Check sheet for the modelled part. Datum: model origin and axes. Units: mm. A direction names the side the tool comes from. Round coordinates to 2 decimals unless told otherwise and drop trailing zeros. Loops run counter-clockwise (first coordinate to the right, second up) from the corner with the lowest first, then second, coordinate; pieces in that order, holes last. Notation, with made-up numbers: (-24.5, 0) -> (16.5, 0) arc R14 ccw to (16.5, 5) -> close; hole circle Ø11 at (-1, -12.75). An arc over 180 degrees is marked (long way). One line per question, with ' | ' between items.
```python
from build123d import *

# Parameters (mm, degrees)
ESQUISSE1_W                  = 16.3
ESQUISSE1_H                  = 12
BOSS_EXTRU_1_DEPTH           = 10.7
ENL_V_MAT_EXTRU_1_DEPTH      = 9
ESQUISSE4_W                  = 5.6
ESQUISSE4_H                  = 3.1
BOSS_EXTRU_2_DEPTH           = 8.8
CHANFREIN1_SIZE              = 0.2
CONG_1_R                     = 0.1
ESQUISSE5_W                  = 1.55
ESQUISSE5_H                  = 0.3
BOSS_EXTRU_3_DEPTH           = 4.3
BOSS_EXTRU_4_DEPTH           = 2.6
BOSS_EXTRU_4_DRAFT           = -15
BOSS_EXTRU_4_PROFILE_2_DEPTH = 2.6
BOSS_EXTRU_4_PROFILE_2_DRAFT = -15
CONG_3_R                     = 0.15


with BuildPart() as part:
    # Esquisse1 → Boss.-Extru.1 (new body)
    with BuildSketch(Plane(origin=(0, 0, 0), x_dir=(1, 0, 0), z_dir=(0, 1, 0))):
        with Locations((-8.15, 6)):
            Rectangle(ESQUISSE1_W, ESQUISSE1_H)
    extrude(amount=BOSS_EXTRU_1_DEPTH)

    # Esquisse2 → Enlèv. mat.-Extru.1 (cut)
    with BuildSketch(Plane.ZY.offset(16.3)):
        Polygon((-8.6, 9.25), (-10.2, 7.65), (-10.2, 1.65), (-1.8, 1.65), (-1.8, 7.65), (-3.4, 9.25), align=None)
    extrude(amount=-ENL_V_MAT_EXTRU_1_DEPTH, mode=Mode.SUBTRACT)

    # Esquisse4 → Boss.-Extru.2 (add)
    with BuildSketch(Plane.ZY.offset(7.3)):
        with Locations((-6, 5.4)):
            Rectangle(ESQUISSE4_W, ESQUISSE4_H)
    extrude(amount=BOSS_EXTRU_2_DEPTH)

    # Chanfrein1
    chanfrein1_edges = [part.edges().sort_by_distance(p)[0] for p in [
        (-16.3, 4.65, -10.2),
        (-16.3, 1.65, -6),
        (-16.3, 4.65, -1.8),
        (-16.3, 8.45, -2.6),
        (-16.3, 9.25, -6),
        (-16.3, 8.45, -9.4),
        (-11.7, 6.95, -8.8),
        (-11.7, 3.85, -8.8),
        (-11.7, 3.85, -3.2),
        (-11.7, 6.95, -3.2),
        (-16.1, 5.4, -8.8),
        (-16.1, 3.85, -6),
        (-16.1, 5.4, -3.2),
        (-16.1, 6.95, -6),
    ]]
    chamfer(chanfrein1_edges, length=CHANFREIN1_SIZE)

    # Congé1
    cong_1_edges = [part.edges().sort_by_distance(p)[0] for p in [
        (-16.3, 10.7, -6),
        (-8.15, 10.7, 0),
        (-16.3, 0, -6),
        (-8.15, 10.7, -12),
        (-16.3, 5.35, 0),
        (-16.3, 5.35, -12),
    ]]
    fillet(cong_1_edges, radius=CONG_1_R)

    # Esquisse5 → Boss.-Extru.3 (add)
    with BuildSketch(Plane.XZ):
        with Locations((-6.025, -0.15)):
            Rectangle(ESQUISSE5_W, ESQUISSE5_H)
        with Locations((-6.025, -11.85)):
            Rectangle(ESQUISSE5_W, ESQUISSE5_H)
    extrude(amount=BOSS_EXTRU_3_DEPTH)


with BuildPart() as boss_extru_4_tool:
    # Esquisse6 → Boss.-Extru.4 (with draft: the straight prism first)
    with BuildSketch(Plane(origin=(0, -1.55, 0), x_dir=(1, 0, 0), z_dir=(0, 1, 0))):
        with BuildLine():
            ThreePointArc((-6.8, 0.85), (-7.5, 0.15), (-6.8, -0.55))
            Line((-6.8, -0.55), (-5.25, -0.55))
            ThreePointArc((-5.25, -0.55), (-4.55, 0.15), (-5.25, 0.85))
            Line((-5.25, 0.85), (-6.8, 0.85))
        make_face()
    extrude(amount=-BOSS_EXTRU_4_DEPTH)
    # Boss.-Extru.4: the draft: its side faces are tilted about the plane it starts from
    boss_extru_4_sides = [boss_extru_4_tool.faces().sort_by_distance(p)[0] for p in [
        (-6.025, -2.85, 0.55),
        (-4.55, -2.85, -0.15),
        (-6.025, -2.85, -0.85),
        (-7.5, -2.85, -0.15),
    ]]
    draft(boss_extru_4_sides, Plane(origin=(0, -1.55, 0), x_dir=(1, 0, 0), z_dir=(0, 1, 0)), BOSS_EXTRU_4_DRAFT)


with BuildPart() as part_1:
    add(part.part)

    # Boss.-Extru.4: add boss_extru_4_tool
    add(boss_extru_4_tool.part)


with BuildPart() as boss_extru_4_profile_2_tool:
    # Esquisse6 → Boss.-Extru.4 profile 2 (with draft: the straight prism first)
    with BuildSketch(Plane(origin=(0, -1.55, 0), x_dir=(1, 0, 0), z_dir=(0, 1, 0))):
        with BuildLine():
            ThreePointArc((-6.8, 12.55), (-7.5, 11.85), (-6.8, 11.15))
            Line((-6.8, 11.15), (-5.25, 11.15))
            ThreePointArc((-5.25, 11.15), (-4.55, 11.85), (-5.25, 12.55))
            Line((-5.25, 12.55), (-6.8, 12.55))
        make_face()
    extrude(amount=-BOSS_EXTRU_4_PROFILE_2_DEPTH)
    # Boss.-Extru.4 profile 2: the draft: its side faces are tilted about the plane it starts from
    boss_extru_4_profile_2_sides = [boss_extru_4_profile_2_tool.faces().sort_by_distance(p)[0] for p in [
        (-7.5, -2.85, -11.85),
        (-6.025, -2.85, -11.15),
        (-4.55, -2.85, -11.85),
        (-6.025, -2.85, -12.55),
    ]]
    draft(boss_extru_4_profile_2_sides, Plane(origin=(0, -1.55, 0), x_dir=(1, 0, 0), z_dir=(0, 1, 0)), BOSS_EXTRU_4_PROFILE_2_DRAFT)


with BuildPart() as part_2:
    add(part_1.part)

    # Boss.-Extru.4 profile 2: add boss_extru_4_profile_2_tool
    add(boss_extru_4_profile_2_tool.part)

    # Congé3
    cong_3_edges = [part_2.edges().sort_by_distance(p)[0] for p in [
        (-6.8, -4.3, -0.15),
        (-6.025, -4.3, -0.3),
        (-5.25, -4.3, -0.15),
        (-6.025, -4.3, 0),
        (-6.025, -4.3, -12),
        (-5.25, -4.3, -11.85),
        (-6.025, -4.3, -11.7),
        (-6.8, -4.3, -11.85),
    ]]
    fillet(cong_3_edges, radius=CONG_3_R - 0.0001)  # a hair under: the kernel refuses the full size


solid = part_2.part
```
(1) Set-up check for faces 4 (the face through (-6.04, -2.56, -11.42)), 5 (the face through (-8, 4, -12)), 6 (the face through (-8, 10.7, -6)), 7 (the face through (-4.894, -2.832, -0.142)), 8 (the face through (-11.76, 8.44, -2.59)): record each of +Z, -Z, +X, -X, +Y, -Y from which the full face is reachable in a straight line by a thin tool's end or side.
Answer:
face 4: +X, -X, -Y | face 5: -Z, +X, -X, +Y | face 6: +Z, -Z, +X, -X, +Y | face 7: +X, -Y | face 8: -X
(2) Go/stop test with flat-tipped pins: pin 1 (6.5 mm diameter, centred on x = -9.5, y = 5, fed in from +Z); pin 2 (6 mm diameter, centred on x = -5, z = -6, fed in from -Y); pin 3 (3 mm diameter, centred on y = 5.5, z = -7, fed in from -X). Record where each tip stops, or that it passes through.
Answer:
pin 1: stops at z = 0 | pin 2: stops at y = 0 | pin 3: stops at x = -16.1
(3) Scan lines: probe 1 along Y at (x, z) = (-14, -6.5); probe 2 along Z at (x, y) = (-15.5, 3.25). Record each from-to range of solid material in increasing order.
Answer:
probe 1: y = 0 to 1.65, 3.85 to 6.95, 9.25 to 10.7 | probe 2: z = -12 to -10.2, -1.8 to 0
(4) Sectioned sample at B-B, the plane x = -3. Record the cut outline in (y, z).
Answer:
outline: (0, -12) -> (10.6, -12) arc R0.1 ccw to (10.7, -11.9) -> (10.7, -0.1) arc R0.1 ccw to (10.6, 0) -> (0, 0) -> close
(5) Sectioned sample at A-A, the plane z = -8.25. Record the cut outline in (x, y).
Answer:
outline: (-16.3, 0.1) arc R0.1 ccw to (-16.2, 0) -> (0, 0) -> (0, 10.7) -> (-16.2, 10.7) arc R0.1 ccw to (-16.3, 10.6) -> (-16.3, 9.45) -> (-16.1, 9.25) -> (-7.3, 9.25) -> (-7.3, 6.95) -> (-15.9, 6.95) -> (-16.1, 6.75) -> (-16.1, 4.05) -> (-15.9, 3.85) -> (-7.3, 3.85) -> (-7.3, 1.65) -> (-16.1, 1.65) -> (-16.3, 1.45) -> close
(6) Mould release check, pull along Y, two halves, no side actions. Record for faces 1 (the face through (-6.01, -2.56, -12.28)), 2 (the face through (-12, 6.95, -6)), 3 (the face through (-8, 4, 0)): +Y half, -Y half, draft (parallel to the pull), parting line (faces both ways), or undercut.
Answer:
face 1: -Y half | face 2: undercut | face 3: draft
(7) Sectioned sample at C-C, the plane z = -2.75. Record the cut outline in (x, y), and give its area (3 significant figures).
Answer:
outline: (-16.3, 0.1) arc R0.1 ccw to (-16.2, 0) -> (0, 0) -> (0, 10.7) -> (-16.2, 10.7) arc R0.1 ccw to (-16.3, 10.6) -> (-16.3, 8.88) -> (-16.1, 8.6) -> (-7.3, 8.6) -> (-7.3, 1.65) -> (-16.1, 1.65) -> (-16.3, 1.45) -> close | area: 112 mm2
